Geometry: final body of the model. Coordinates: model frame, mm. Round coordinates to 2 decimals unless told otherwise and drop trailing zeros. Loops run counter-clockwise (first coordinate to the right, second up) from the corner with the lowest first, then second, coordinate; pieces in that order, holes last. Notation, with made-up numbers: M 57,9.25 L 115,9.25 A35 ccw 115,42.25 Z; hole C 24,-4.5 d2. An arc over 180 degrees is marked long. Write each question's results on one line, items separated by ' | '.
```python
from build123d import *

# Parameters (mm, degrees)
F0_R     = 82.559423
F0_R_2   = 4.557666
F1_DEPTH = 635
F2_R     = 6
F3_SIZE  = 6


with BuildPart() as f1:
    # F0 (on Front) → F1 (new body, symmetric)
    with BuildSketch(Plane.XZ):
        Circle(F0_R)
        Circle(F0_R_2, mode=Mode.SUBTRACT)
    extrude(amount=F1_DEPTH, both=True)

    # F2
    f2_edges = [f1.edges().sort_by_distance(p)[0] for p in [
        (-82.559423, 635, 0),
        (-4.557666, 635, 0),
    ]]
    fillet(f2_edges, radius=F2_R)

    # F3
    f3_edges = [f1.edges().sort_by_distance(p)[0] for p in [
        (-82.559423, -635, 0),
    ]]
    chamfer(f3_edges, length=F3_SIZE)


solid = f1.part
```
1. Draft query along X for faces 1 (the face through (-1, 635, -16)), 2 (the face through (73.3, -634.71, 23.08)). Return one class per face: pulls with the +X half, pulls with the -X half, needs draft (parallel to the pull), parting line crosses it, or undercut.
Answer key:
face 1: needs draft | face 2: parting line crosses it
2. Section A-A (y = 222). Output: boundary loops of the cut face in (x, z), then the cut area to 3 significant figures.
Answer key:
outline: C 0,0 d165.12; hole C 0,0 d9.12 | area: 21,300 mm²
3. Ray query, probe 1 along Z at (x, y) = (0, -34); probe 2 along Z at (x, y) = (-1.5, 239.5); probe 3 along Y at (x, z) = (63, -43.5). Return the intervals inside material, ascending.
Answer key:
probe 1: z = -82.56 to -4.56, 4.56 to 82.56 | probe 2: z = -82.55 to -4.3, 4.3 to 82.55 | probe 3: y = -635 to 635
4. Pin query (flat end, axial travel): P1, Ø3, axis at x = 5.5, y = -110.5, coming from the +Z side; P2, Ø2, axis at x = 20.5, y = -404.5, coming from the +Z side; P3, Ø2, axis at x = -30, y = -155.5, coming from the -Z side. Return the tip coordinate at first contact, or that it passes through.
Answer key:
P1: stops at z = 82.46 | P2: stops at z = 80.22 | P3: stops at z = -77.3
